Here's how the part is built. I have some questions about the finished solid (model axes, mm). A direction names the side the tool comes from. Coordinates: 2 decimals unless noted, no trailing zeros. Loops run counter-clockwise (first coordinate to the right, second up) from the corner with the lowest first, then second, coordinate; pieces in that order, holes last. Notation, with made-up numbers: (25, 54) -> (43, 54) arc R15 cw to (43, 74) -> close; hole circle Ø8 at (39.25, -35). An arc over 180 degrees is marked (long way). Answer as a JSON object with one key per item and string values. Group by question number.
1) Which directions (+Z, -Z, +X, -X, +Y, -Y) give clear straight access to the entire face, cutting with the end or side of a thin tool? Please do faces 1 (the flat face through (-14.64, 1.52, 59.99)), 2 (the flat face through (82, 0, 42)).
2) I want a section at A-A (z = -134). Write out the boundary of the cut face in (x, y).
3) I need wall thicknesses on probe 1 along Z at (x, y) = (89.5, 2.6); probe 2 along Z at (x, y) = (140, 1.2); probe 3 along X at (y, z) = (1.1, 38). Which ranges of each line are inside material? Lowest first, please. Write a range as [from, to].
4) If we mould it in two halves opening along X, with no side actions, what happens to faces 3 (the cylindrical face through (31.617, 1.521, 132.977)), 4 (the flat face through (82, 3, 42))? For each: +X half, -X half, draft (parallel to the pull), parting line (faces both ways), or undercut.
5) I want a section at B-B (z = -24). Write out the boundary of the cut face in (x, y).
6) I'm going to push flat-ended pins straight in: pin 1 (1.5 mm diameter, centred on x = 102.5, y = 2, fed in from +Z); pin 2 (1.5 mm diameter, centred on x = -48.5, y = 1, fed in from -Z). Where does each tip first touch, or does it pass through?
7) I want a section at C-C (y = 0.55). Count the separate pieces of the cut face and the enclosed holes in it, then the cut area to 3 significant figures.
```python
from build123d import *

# Parameters (mm, degrees)
SKETCH_1_W           = 240
SKETCH_1_H           = 400
EXTRUDE_1_DEPTH      = 3
SKETCH_9_W           = 10
SKETCH_9_H           = 3
SKETCH_9_W_2         = 20
SKETCH_9_W_3         = 15
EXTRUDE_2_DEPTH      = 3
SKETCH_13_W          = 10
SKETCH_13_H          = 3
CUT_EXTRUDE_1_DEPTH  = 3
SKETCH_12_R          = 2.5
CUT_EXTRUDE_2_DEPTH  = 3
SKETCH_10_R          = 2.5
CUT_EXTRUDE_3_DEPTH  = 3
SKETCH_14_R          = 1.6
CUT_EXTRUDE_4_DEPTH  = 3
SKETCH_23_R          = 1.5
CUT_EXTRUDE_11_DEPTH = 10
SKETCH_21_W          = 22.5
SKETCH_21_H          = 30.5
CUT_EXTRUDE_12_DEPTH = 10
SKETCH_24_R          = 1.625
CUT_EXTRUDE_13_DEPTH = 10


with BuildPart() as part:
    # 草图1 → 凸台-拉伸1 (new body)
    with BuildSketch(Plane(origin=(46.742818835, 0, -86.416508262), x_dir=(1, 0, 0), z_dir=(0, 1, 0))):
        with Locations((-16.707557602, -86.429149101)):
            Rectangle(SKETCH_1_W, SKETCH_1_H)
    extrude(amount=EXTRUDE_1_DEPTH)

    # 草图9 → 凸台-拉伸2 (add)
    with BuildSketch(Plane(origin=(0, 3, 0), x_dir=(1, 0, 0), z_dir=(0, 1, 0))):
        with Locations((145.035261234, -201.512640839)):
            Rectangle(SKETCH_9_W, SKETCH_9_H)
        with Locations((120.035261234, -201.512640839)):
            Rectangle(SKETCH_9_W_2, SKETCH_9_H)
        with Locations((95.035261234, -201.512640839)):
            Rectangle(SKETCH_9_W, SKETCH_9_H)
        with Locations((145.035261234, 201.487359161)):
            Rectangle(SKETCH_9_W, SKETCH_9_H)
        with Locations((120.035261234, 201.487359161)):
            Rectangle(SKETCH_9_W_2, SKETCH_9_H)
        with Locations((95.035261234, 201.487359161)):
            Rectangle(SKETCH_9_W, SKETCH_9_H)
        with Locations((-57.464738766, 201.487359161)):
            Rectangle(SKETCH_9_W_3, SKETCH_9_H)
        with Locations((-82.464738766, -201.512640839)):
            Rectangle(SKETCH_9_W_3, SKETCH_9_H)
        with Locations((-57.464738766, -201.512640839)):
            Rectangle(SKETCH_9_W_3, SKETCH_9_H)
        with Locations((-82.464738766, 201.487359161)):
            Rectangle(SKETCH_9_W_3, SKETCH_9_H)
    extrude(amount=-EXTRUDE_2_DEPTH)

    # 草图13 → 切除-拉伸1 (cut)
    with BuildSketch(Plane(origin=(0, 3, 0), x_dir=(1, 0, 0), z_dir=(0, 1, 0))):
        with Locations((135.035261234, -183.512640839)):
            Rectangle(SKETCH_13_W, SKETCH_13_H)
        with Locations((105.035261234, -183.512640839)):
            Rectangle(SKETCH_13_W, SKETCH_13_H)
        with Locations((135.035261234, 183.487359161)):
            Rectangle(SKETCH_13_W, SKETCH_13_H)
        with Locations((105.035261234, 183.487359161)):
            Rectangle(SKETCH_13_W, SKETCH_13_H)
    extrude(amount=-CUT_EXTRUDE_1_DEPTH, mode=Mode.SUBTRACT)

    # 草图12 → 切除-拉伸2 (cut)
    with BuildSketch(Plane(origin=(0, 3, 0), x_dir=(1, 0, 0), z_dir=(0, 1, 0))):
        with Locations(Location((-82.464738766, -120.012640839, 0), (0, 0, 270))):
            Circle(SKETCH_12_R)
        with Locations(Location((-82.464738766, -40.012640839, 0), (0, 0, 270))):
            Circle(SKETCH_12_R)
        with Locations(Location((-82.464738766, 119.987359161, 0), (0, 0, 270))):
            Circle(SKETCH_12_R)
        with Locations(Location((-82.464738766, 39.987359161, 0), (0, 0, 270))):
            Circle(SKETCH_12_R)
    extrude(amount=-CUT_EXTRUDE_2_DEPTH, mode=Mode.SUBTRACT)

    # 草图10 → 切除-拉伸3 (cut)
    with BuildSketch(Plane(origin=(0, 3, 0), x_dir=(1, 0, 0), z_dir=(0, 1, 0))):
        with Locations(Location((50.035261234, -192.512640839, 0), (0, 0, 270))):
            Circle(SKETCH_10_R)
        with Locations(Location((10.035261234, -192.512640839, 0), (0, 0, 270))):
            Circle(SKETCH_10_R)
        with Locations(Location((50.055539801, 192.497892125, 0), (0, 0, 90))):
            Circle(SKETCH_10_R)
        with Locations(Location((10.055540023, 192.502105738, 0), (0, 0, 90))):
            Circle(SKETCH_10_R)
    extrude(amount=-CUT_EXTRUDE_3_DEPTH, mode=Mode.SUBTRACT)

    # 草图14 → 切除-拉伸4 (cut)
    with BuildSketch(Plane(origin=(0, 3, 0), x_dir=(1, 0, 0), z_dir=(0, 1, 0))):
        with Locations(Location((90.035261234, -34.012640839, 0), (0, 0, 270))):
            Circle(SKETCH_14_R)
        with Locations(Location((-29.964738766, -34.012640839, 0), (0, 0, 90))):
            Circle(SKETCH_14_R)
        with Locations(Location((90.035261234, -128.012640839, 0), (0, 0, 270))):
            Circle(SKETCH_14_R)
        with Locations(Location((-29.964738766, -128.012640839, 0), (0, 0, 90))):
            Circle(SKETCH_14_R)
        with Locations(Location((-29.964738766, 59.987359161, 0), (0, 0, 270))):
            Circle(SKETCH_14_R)
        with Locations(Location((90.035261234, 59.987359161, 0), (0, 0, 90))):
            Circle(SKETCH_14_R)
        with BuildLine():
            Line((-4.071414156, -105.869783696), (-25.509895829, -12.808559206))
            ThreePointArc((-25.509895829, -12.808559206), (28.551489229, 56.968043789), (86.171099154, -9.900395941))
            Line((86.171099154, -9.900395941), (64.504635396, -104.08406941))
            ThreePointArc((64.504635396, -104.08406941), (30.946349307, -133.000780522), (-4.071414156, -105.869783696))
        make_face()
    extrude(amount=-CUT_EXTRUDE_4_DEPTH, mode=Mode.SUBTRACT)

    # 草图23 → 切除-拉伸11 (cut)
    with BuildSketch(Plane(origin=(0, 3, 0), x_dir=(1, 0, 0), z_dir=(0, 1, 0))):
        with Locations(Location((-18.714738766, 170.487359161, 0), (0, 0, 270))):
            Circle(SKETCH_23_R)
        with Locations(Location((25.785261234, 125.987359161, 0), (0, 0, 270))):
            Circle(SKETCH_23_R)
        with Locations(Location((-18.714738766, 81.487359161, 0), (0, 0, 270))):
            Circle(SKETCH_23_R)
        with Locations(Location((-63.214738766, 125.987359161, 0), (0, 0, 270))):
            Circle(SKETCH_23_R)
        with BuildLine():
            Line((-58.714738766, 125.987359161), (-58.714738766, 85.987359161))
            Line((-58.714738766, 85.987359161), (-18.714738766, 85.987359161))
            ThreePointArc((-18.714738766, 85.987359161), (9.569532481, 154.271630409), (-58.714738766, 125.987359161))
        make_face()
    extrude(amount=-CUT_EXTRUDE_11_DEPTH, mode=Mode.SUBTRACT)

    # 草图21 → 切除-拉伸12 (cut)
    with BuildSketch(Plane(origin=(0, 3, 0), x_dir=(1, 0, 0), z_dir=(0, 1, 0))):
        with Locations((-49.214738766, -0.012640839)):
            Rectangle(SKETCH_21_W, SKETCH_21_H)
    extrude(amount=-CUT_EXTRUDE_12_DEPTH, mode=Mode.SUBTRACT)

    # 草图24 → 切除-拉伸13 (cut)
    with BuildSketch(Plane.XZ):
        with Locations(Location((-37.964738766, -179.987359161, 0), (0, 0, 270))):
            Circle(SKETCH_24_R)
        with Locations(Location((-17.964738766, -179.987359161, 0), (0, 0, 270))):
            Circle(SKETCH_24_R)
        with Locations(Location((90.035261234, -179.987359161, 0), (0, 0, 270))):
            Circle(SKETCH_24_R)
        with Locations(Location((70.035261234, -179.987359161, 0), (0, 0, 270))):
            Circle(SKETCH_24_R)
    extrude(amount=-CUT_EXTRUDE_13_DEPTH, mode=Mode.SUBTRACT)


solid = part.part
```
Determined:
{
 "1": {"face 1": "+Y, -Y", "face 2": "+Z, -Z, +X, -X, -Y"},
 "2": {"outline": "(-89.96, 0) -> (-57.9, 0) -> (-57.9, 3) -> (-89.96, 3) -> close; (20.47, 0) -> (150.04, 0) -> (150.04, 3) -> (20.47, 3) -> close"},
 "3": {"probe 1": "[-199.99, -181.52], [-178.45, -61.5], [-58.48, 32.5], [35.52, 126.5], [129.52, 200.01]", "probe 2": "[-199.99, -184.99], [-181.99, 182.01], [185.01, 200.01]", "probe 3": "[-89.96, -83.95], [-80.98, -19.71], [79.71, 150.04]"},
 "4": {"face 3": "undercut", "face 4": "draft"},
 "5": {"outline": "(-89.96, 0) -> (-21.66, 0) -> (-21.66, 3) -> (-89.96, 3) -> close; (81.73, 0) -> (150.04, 0) -> (150.04, 3) -> (81.73, 3) -> close"},
 "6": {"pin 1": "z = 200.01", "pin 2": "z = -199.99"},
 "7": {"separate pieces": "1", "enclosed holes": "29", "area": "73,700 mm^2"}
}
